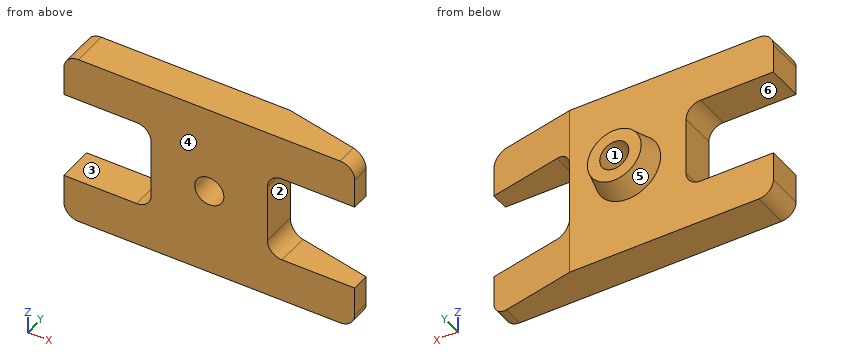
from build123d import *

# Parameters (mm, degrees)
SKETCH1_W               = 200
SKETCH1_H               = 120
SKETCH1_R               = 22.5
BOSS_EXTRUDE1_DEPTH     = 25
SKETCH1_3_R             = 22.5
BOSS_EXTRUDE2_DEPTH     = 40
SKETCH2_R               = 10
CUT_EXTRUDE1_DEPTH      = 124.288280059
FILLET1_R               = 10
SKETCH3_W               = 60
SKETCH3_H               = 60
CUT_EXTRUDE2_DEPTH      = 120.268604419
FILLET2_R               = 10
CUT_EXTRUDE3_DEPTH      = 124.288280059
CUT_EXTRUDE3_DEPTH_BACK = 124.288280059


# Read off the part's stored shape, not the designer's step: Draft1
with BuildPart() as part:
    # Sketch1 → Boss-Extrude1 (new body)
    with BuildSketch(Plane(origin=(0, 0, 0), x_dir=(1, 0, 0), z_dir=(0, 1, 0))):
        Rectangle(SKETCH1_W, SKETCH1_H)
        with Locations(Location((0, 0, 0), (0, 0, 270))):
            Circle(SKETCH1_R, mode=Mode.SUBTRACT)
    extrude(amount=BOSS_EXTRUDE1_DEPTH)

    # Sketch1<3> → Boss-Extrude2 (add)
    with BuildSketch(Plane(origin=(0, 0, 0), x_dir=(1, 0, 0), z_dir=(0, 1, 0))):
        with Locations(Location((0, 0, 0), (0, 0, 270))):
            Circle(SKETCH1_3_R)
    extrude(amount=BOSS_EXTRUDE2_DEPTH)

    # Draft1 outline → Draft1 (revolve, cut)
    with BuildSketch(Plane.XY):
        Polygon((22.5, 40), (18.480762114, 40), (22.5, 25), align=None)
    revolve(axis=Axis((0, 0, 0), (0, 1, 0)), mode=Mode.SUBTRACT)

    # Sketch2 → Cut-Extrude1 (cut, through all)
    with BuildSketch(Plane(origin=(0, 40, 0), x_dir=(1, 0, 0), z_dir=(0, 1, 0))):
        with Locations(Location((0, 0, 0), (0, 0, 270))):
            Circle(SKETCH2_R)
    extrude(amount=-CUT_EXTRUDE1_DEPTH, mode=Mode.SUBTRACT)

    # Fillet1
    fillet1_edges = [part.edges().sort_by_distance(p)[0] for p in [
        (-100, 12.5, -60),
        (100, 12.5, -60),
        (100, 12.5, 60),
        (-100, 12.5, 60),
    ]]
    fillet(fillet1_edges, radius=FILLET1_R)

    # Sketch3 → Cut-Extrude2 (cut, through all)
    with BuildSketch(Plane(origin=(0, 25, 0), x_dir=(1, 0, 0), z_dir=(0, 1, 0))):
        with Locations((-70, 0)):
            Rectangle(SKETCH3_W, SKETCH3_H)
        with Locations((70, 0)):
            Rectangle(SKETCH3_W, SKETCH3_H)
    extrude(amount=-CUT_EXTRUDE2_DEPTH, mode=Mode.SUBTRACT)

    # Fillet2
    fillet2_edges = [part.edges().sort_by_distance(p)[0] for p in [
        (-40, 12.5, -30),
        (-40, 12.5, 30),
        (40, 12.5, -30),
        (40, 12.5, 30),
    ]]
    fillet(fillet2_edges, radius=FILLET2_R)

    # Sketch4 → Cut-Extrude3 (cut, two sides: drawn at the far end of the back side and taken through both)
    with BuildSketch(Plane.XY.offset(-CUT_EXTRUDE3_DEPTH_BACK)):
        Polygon((40, 25), (100, 12.5), (100, 25), align=None)
    extrude(amount=CUT_EXTRUDE3_DEPTH + CUT_EXTRUDE3_DEPTH_BACK, mode=Mode.SUBTRACT)


solid = part.part
The model under review builds one solid part; all positions refer to its coordinate system, in mm. Face numbers are marked on the shaded views. A direction names the side the tool comes from. Round coordinates to 2 decimals unless told otherwise and drop trailing zeros. Write each loop counter-clockwise with the first axis right and the second up, starting at its lowest first coordinate (ties: lowest second). Pieces come first, ordered by that corner, then holes. Notation, with made-up numbers: (41, -8) - (65, -8) arc R10 cw to (65, 6) - close; hole circle Ø11 at (1, 12). An arc over 180 degrees is marked (long way). One line per item, written item: value. Start each with the question number.
1. Consider section B-B on x = -53. Write out the cut boundary in (y, z).
2. Clearance check with flat-ended pins moving along their axes: P1, Ø6, axis at x = 18, z = -23, coming from the +Y side; P2, Ø12.5, axis at y = 18.5, z = -1.5, coming from the +X side; P3, Ø1, axis at y = 15, z = -11.5, coming from the -X side. State where each tip first meets the part, or that it passes through.
3. Consider section C-C on y = 4. Write out the cut boundary in (x, z).
4. Consider section A-A on z = 0. Write out the cut boundary in (x, y), and give its area (3 significant figures).
5. The part is to be moulded in two halves that separate along Z. For the marked faces 4, 5 and 6, say which applies: released by +Z, released by -Z, zero draft, split by the parting line, or undercut.
6. Machinability: for the marked faces 1, 2 and 3, which of the approach directions +Z, -Z, +X, -X, +Y, -Y give a long, thin tool a straight path to every point of the face, cutting with its end or side? Answer none if there is none.
7. To check wall thickness, follow L1, parallel to Z at x = 88, y = 9; L2, parallel to X at y = 15, z = 0; L3, parallel to Y at x = -17.5, z = 19. State the ranges of each line that lie inside material, in increasing order. Write a range as from..to.
8. Consider section D-D on z = -34. Write out the cut boundary in (x, y), and give its area (4 significant figures).
Checks:
1. outline: (0, -60) - (25, -60) - (25, -30) - (0, -30) - close; (0, 30) - (25, 30) - (25, 60) - (0, 60) - close
2. P1: stops at y = 25
2. P2: stops at x = 40
2. P3: stops at x = -40
3. outline: (-100, -50) arc R10 ccw to (-90, -60) - (90, -60) arc R10 ccw to (100, -50) - (100, -30) - (50, -30) arc R10 cw to (40, -20) - (40, 20) arc R10 cw to (50, 30) - (100, 30) - (100, 50) arc R10 ccw to (90, 60) - (-90, 60) arc R10 ccw to (-100, 50) - (-100, 30) - (-50, 30) arc R10 cw to (-40, 20) - (-40, -20) arc R10 cw to (-50, -30) - (-100, -30) - close; hole circle Ø20 at (0, 0)
4. outline: (-40, 0) - (-10, 0) - (-10, 40) - (-18.48, 40) - (-22.5, 25) - (-40, 25) - close; (10, 0) - (40, 0) - (40, 25) - (22.5, 25) - (18.48, 40) - (10, 40) - close
4. area: 1,810 mm^2
5. face 4: zero draft
5. face 5: split by the parting line
5. face 6: undercut
6. face 1: +Y, -Y
6. face 2: +X, +Y, -Y
6. face 3: -X, +Y, -Y
7. L1: z = -60..-30, 30..60
7. L2: x = -40..-10, 10..40
7. L3: y = 0..25
8. outline: (-100, 0) - (100, 0) - (100, 12.5) - (40, 25) - (-100, 25) - close
8. area: 4,625 mm^2
